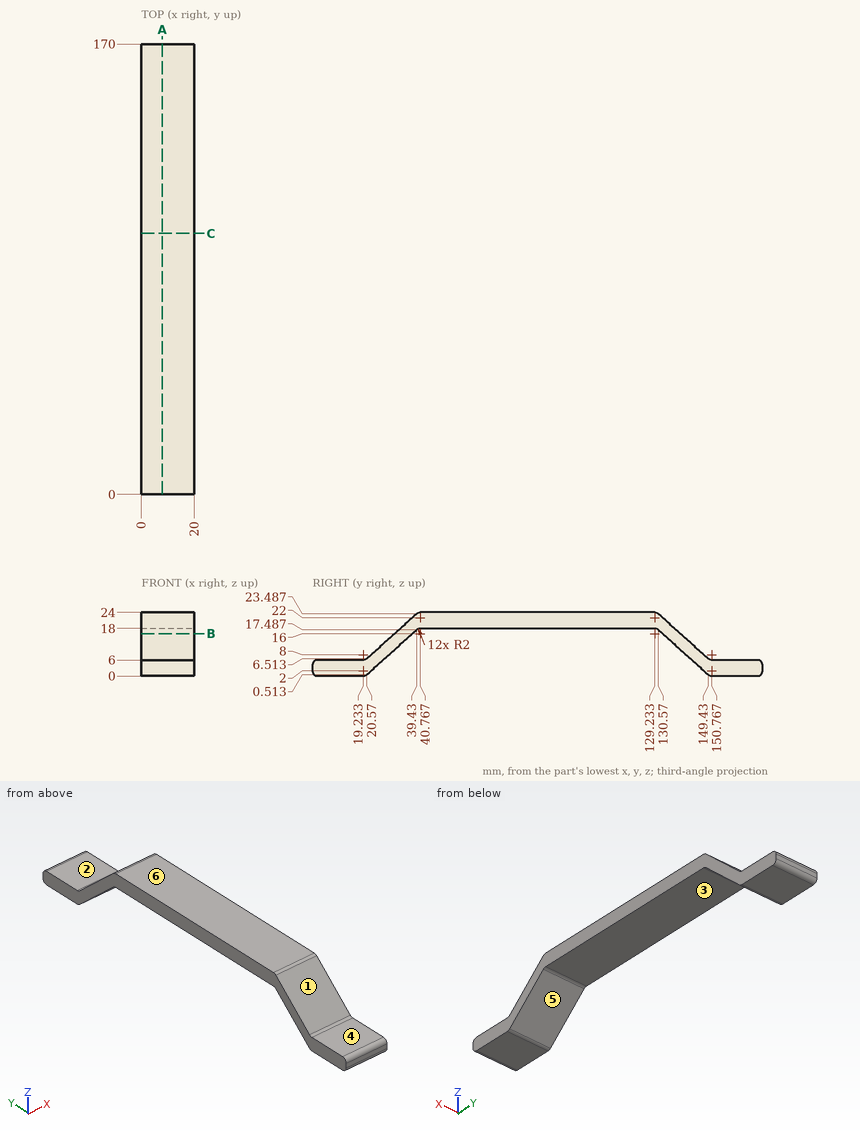
Geometry: see drawing. Coordinates: mm, zero at the bounding-box minimum. A direction names the side the tool comes from. Round coordinates to 2 decimals unless told otherwise and drop trailing zeros. Write each loop counter-clockwise with the first axis right and the second up, starting at its lowest first coordinate (ties: lowest second). Pieces come first, ordered by that corner, then holes. Notation, with made-up numbers: (74.25, 34) - (92.25, 34) arc R19 ccw to (92.25, 60) - close; hole circle Ø8 at (78, 81). An arc over 180 degrees is marked (long way). Use CSV: the item, a comma, the result in double quotes. Start each with the question number.
(1) Cut plane B-B, the plane z = 16. Return loops of the section in (x, y), and give its area (3 significant figures).
(2) Material intervals for probe 1 along Z at (x, y) = (2.25, 120); probe 2 along Y at (x, z) = (15, 8.25) (1 decimal); probe 3 along Y at (x, z) = (15.75, 1.75) (1 decimal), sorted ascending. Write a range as [from, to].
(3) First-contact query: pin 1 Ø8.5 at (x, y) = (10, 158.5) entering from +Z; pin 2 Ø12 at (x, y) = (9.5, 140) entering from -Z; pin 3 Ø8 at (x, y) = (4.5, 30.5) entering from -Z. Flat tips, straight axial feed; report the tip coordinate or a pass-through.
(4) Mould query, pull axis Y, two halves, no side actions, for the marked faces 1, 2 and 3. Classes: pulls with the +Y half, pulls with the -Y half, needs draft (parallel to the pull), parting line crosses it, or undercut.
(5) Set-up query: the marked faces 4, 5 and 6. Return all of +Z, -Z, +X, -X, +Y, -Y with unobstructed straight access to the full face (end or side cutting, diameter ignored); none if empty.
(6) Cut plane C-C, the plane y = 98.5. Return loops of the section in (x, z), and give its area (3 significant figures).
(7) Cut plane A-A, the plane x = 8. Return loops of the section in (y, z), and give its area (3 significant figures).
Geometry says:
1,outline,"(0, 31.11) - (20, 31.11) - (20, 37.78) - (0, 37.78) - close; (0, 132.22) - (20, 132.22) - (20, 138.89) - (0, 138.89) - close"
1,area,"267 mm²"
2,probe 1,"[18, 24]"
2,probe 2,"[22.5, 29.2], [140.8, 147.5]"
2,probe 3,"[0, 21.9], [148.1, 170]"
3,pin 1,"z = 6"
3,pin 2,"z = 3.6"
3,pin 3,"z = 5.85"
4,face 1,"pulls with the -Y half"
4,face 2,"needs draft"
4,face 3,"undercut"
5,face 4,"+Z, +X, -X, -Y"
5,face 5,"-Z, +X, -X"
5,face 6,"+Z, +X, -X, +Y, -Y"
6,outline,"(0, 18) - (20, 18) - (20, 24) - (0, 24) - close"
6,area,"120 mm²"
7,outline,"(0, 2) arc R2 ccw to (2, 0) - (19.23, 0) arc R2 ccw to (20.57, 0.51) - (39.43, 17.49) arc R2 cw to (40.77, 18) - (129.23, 18) arc R2 cw to (130.57, 17.49) - (149.43, 0.51) arc R2 ccw to (150.77, 0) - (168, 0) arc R2 ccw to (170, 2) - (170, 4) arc R2 ccw to (168, 6) - (150.77, 6) arc R2 cw to (149.43, 6.51) - (130.57, 23.49) arc R2 ccw to (129.23, 24) - (40.77, 24) arc R2 ccw to (39.43, 23.49) - (20.57, 6.51) arc R2 cw to (19.23, 6) - (2, 6) arc R2 ccw to (0, 4) - close"
7,area,"1,020 mm²"
